Verification items for the finished model (mm, model axes). A direction names the side the tool comes from. Coordinates: 2 decimals unless noted, no trailing zeros. Order: outer loops, then holes, each group sorted by start corner. A loop starts at its lowest first (then second) coordinate and runs counter-clockwise, first axis right, second up. Notation, with made-up numbers: M 21,0 L 73,0 A15 ccw 73,14 Z; hole C 89,89.5 d3. An arc over 180 degrees is marked long. Write item = value, one per line.
```python
from build123d import *

# Parameters (mm, degrees)
EXTRUDE_577_DEPTH                       = 10
EXTRUDE_START                           = 3
EXTRUDE_1331_DEPTH                      = 2
FILLET_1_R                              = 1
EXTRUDE_2001_DEPTH                      = 6
EXTRUDE_2001_DEPTH_BACK                 = 9
CUT_EXTRUDE_2109_REACH                  = 26.775
CUT_EXTRUDE_2109_END_RADIUS             = 7.25
SKETCH_6_R                              = 1.75
CUT_EXTRUDE_2109_DIRECTION_2_REACH      = 26.775
CUT_EXTRUDE_2109_DIRECTION_2_END_RADIUS = 10.75
SKETCH_7_R                              = 1.4
EXTRUDE_2720_DEPTH                      = 2
EXTRUDE_2720_2_DEPTH                    = 2
CHAMFER_2_SIZE                          = 1.5
EXTRUDE_START_2                         = 1
EXTRUDE_3078_DEPTH                      = 1
CHAMFER_3_SIZE                          = 1.5
CHAMFER_4_SIZE                          = 4.5
CHAMFER_4_SIZE2                         = 0.5


# Some blends are built 0.0001 mm under size
with BuildPart() as part:
    # Эскиз1 → Extrude 577 (new body)
    with BuildSketch(Plane.XY):
        with BuildLine():
            ThreePointArc((-5.712121212, 4.464770012), (0, -7.25), (5.712121212, 4.464770012))
            ThreePointArc((5.712121212, 4.464770012), (5.884169654, 5.868479146), (7.287878788, 5.696430705))
            ThreePointArc((7.287878788, 5.696430705), (0, -9.25), (-7.287878788, 5.696430705))
            ThreePointArc((-7.287878788, 5.696430705), (-5.884169654, 5.868479146), (-5.712121212, 4.464770012))
        make_face()
    extrude(amount=EXTRUDE_577_DEPTH)

    # Эскиз5 → Extrude 2001 (add, two sides: drawn at the far end of the back side and taken through both)
    with BuildSketch(Plane.XY.offset(10).offset(-EXTRUDE_2001_DEPTH_BACK)):
        with BuildLine():
            ThreePointArc((-5.058139535, -5.194008514), (0, -7.25), (5.058139535, -5.194008514))
            ThreePointArc((5.058139535, -5.194008514), (7.532795961, -5.226804475), (7.5, -7.7014609))
            ThreePointArc((7.5, -7.7014609), (0, -10.75), (-7.5, -7.7014609))
            ThreePointArc((-7.5, -7.7014609), (-7.532795961, -5.226804475), (-5.058139535, -5.194008514))
        make_face()
    extrude(amount=EXTRUDE_2001_DEPTH + EXTRUDE_2001_DEPTH_BACK)

    # Cut-Extrude 2109: up to this cylinder (the profile starts outside it)
    cut_extrude_2109_end = Plane(origin=(0, 0, 12), z_dir=(0, 0, -1)) * Cylinder(CUT_EXTRUDE_2109_END_RADIUS, 69.05, mode=Mode.PRIVATE)
    # Эскиз6 → Cut-Extrude 2109 (cut, up to the surface)
    with BuildSketch(Plane(origin=(0, -9.25, 0), x_dir=(-1, 0, 0), z_dir=(0, -1, 0)), mode=Mode.PRIVATE) as cut_extrude_2109_sk1:
        with Locations(Location((0, -12, 0), (0, 0, 270))):
            Circle(SKETCH_6_R)
    cut_extrude_2109_tool1 = extrude(cut_extrude_2109_sk1.sketch, amount=-CUT_EXTRUDE_2109_REACH, mode=Mode.PRIVATE) - cut_extrude_2109_end
    add(cut_extrude_2109_tool1.solids().sort_by_distance((0, -9.25, 12))[0], mode=Mode.SUBTRACT)

    # Cut-Extrude 2109 direction 2: up to this cylinder (the profile starts inside it)
    cut_extrude_2109_direction_2_end = Plane(origin=(0, 0, 12), z_dir=(0, 0, 1)) * Cylinder(CUT_EXTRUDE_2109_DIRECTION_2_END_RADIUS, 76.05, mode=Mode.PRIVATE)
    # Эскиз6 → Cut-Extrude 2109 direction 2 (cut, up to the surface)
    with BuildSketch(Plane(origin=(0, -9.25, 0), x_dir=(-1, 0, 0), z_dir=(0, -1, 0)), mode=Mode.PRIVATE) as cut_extrude_2109_direction_2_sk1:
        with Locations(Location((0, -12, 0), (0, 0, 270))):
            Circle(SKETCH_6_R)
    cut_extrude_2109_direction_2_tool1 = extrude(cut_extrude_2109_direction_2_sk1.sketch, amount=CUT_EXTRUDE_2109_DIRECTION_2_REACH, mode=Mode.PRIVATE) & cut_extrude_2109_direction_2_end
    add(cut_extrude_2109_direction_2_tool1.solids().sort_by_distance((0, -9.25, 12))[0], mode=Mode.SUBTRACT)

    # Фаска2
    chamfer_2_edges = [part.edges().sort_by_distance(p)[0] for p in [
        (-8.027867462, -6.512593205, 1),
        (8.027867462, -6.512593205, 1),
        (0, -10.75, 1),
    ]]
    chamfer(chamfer_2_edges, length=CHAMFER_2_SIZE - 0.0001)  # a hair under: the kernel refuses the full size



with BuildPart() as body_2:
    # Эскиз3 → Extrude 1331 (new body)
    with BuildSketch(Plane(origin=(0, 0, 0), x_dir=(-1, 0, 0), z_dir=(0, 0, -1)).offset(EXTRUDE_START)):
        with BuildLine():
            Line((-1.5, 7.09313048), (-2.75, 0.004028205))
            ThreePointArc((-2.75, 0.004028205), (-3.918577626, -3.728601804), (-6, -7.04006392))
            ThreePointArc((-6, -7.04006392), (0, -9.25), (6, -7.04006392))
            ThreePointArc((6, -7.04006392), (3.918577626, -3.728601804), (2.75, 0.004028205))
            Line((2.75, 0.004028205), (1.5, 7.09313048))
            ThreePointArc((1.5, 7.09313048), (0, 7.25), (-1.5, 7.09313048))
        make_face()
    extrude(amount=-EXTRUDE_1331_DEPTH)

    # Скругление1
    # the kernel refuses this fillet: 1 mm, written as the material it takes off along each edge
    with BuildSketch(Plane(origin=(-17.735965382, 2.646458234, -3), x_dir=(0.6567344577177726, -0.7541219079473445, 0), z_dir=(-0.7541219079473445, -0.6567344577177726, 0))) as fillet_1_piece_1:
        with BuildLine():
            CenterArc((15.217148054 + FILLET_1_R, FILLET_1_R), FILLET_1_R, 180, 90)
            Line((15.217148054 + FILLET_1_R, 0), (15.217148054, 0))
            Line((15.217148054, 0), (15.217148054, FILLET_1_R))
        make_face()
    revolve(axis=Axis((-17.735965382, 2.646458234, -3), (0, 0, 1)), revolution_arc=38.948703068, mode=Mode.SUBTRACT)
    with BuildSketch(Plane(origin=(-2.75, 0.004028205, -3), x_dir=(0, 0, 1), z_dir=(0.17364817766693094, 0.984807753012208, 0)), Plane(origin=(1.065879556, 9.555149862, -3), x_dir=(0, 0, 1), z_dir=(0.1736481776669306, -0.984807753012208, 0))) as fillet_1_piece_2:
        with BuildLine():
            CenterArc((FILLET_1_R, FILLET_1_R), FILLET_1_R, 180, 90)
            Line((0, FILLET_1_R), (0, 0))
            Line((0, 0), (FILLET_1_R, 0))
        make_face()
    extrude(amount=9.698463104, mode=Mode.SUBTRACT)
    with BuildSketch(Plane(origin=(17.735965382, 2.646458234, -3), x_dir=(-0.9848077530122082, -0.17364817766692925, 0), z_dir=(-0.17364817766692925, 0.9848077530122082, 0))) as fillet_1_piece_3:
        with BuildLine():
            CenterArc((15.217148054 + FILLET_1_R, FILLET_1_R), FILLET_1_R, 180, 90)
            Line((15.217148054 + FILLET_1_R, 0), (15.217148054, 0))
            Line((15.217148054, 0), (15.217148054, FILLET_1_R))
        make_face()
    revolve(axis=Axis((17.735965382, 2.646458234, -3), (0, 0, 1)), revolution_arc=38.948703068, mode=Mode.SUBTRACT)


with BuildPart() as body_3:
    # Эскиз7 → Extrude 2720 (new body)
    with BuildSketch(Plane(origin=(0, 0, -3), x_dir=(-1, 0, 0), z_dir=(0, 0, -1))):
        with BuildLine():
            Line((-7.059505235, -8.866162387), (-5.204391621, -7.647013002))
            ThreePointArc((-5.204391621, -7.647013002), (-3.557692308, -8.538461538), (-1.765200931, -9.080009123))
            Line((-1.765200931, -9.080009123), (-1.324605701, -11.255703859))
            ThreePointArc((-1.324605701, -11.255703859), (-6.442307692, -15.461538462), (-7.059505235, -8.866162387))
        make_face()
        with Locations((-5, -12)):
            Circle(SKETCH_7_R, mode=Mode.SUBTRACT)
    extrude(amount=-EXTRUDE_2720_DEPTH)


with BuildPart() as body_4:
    # Эскиз7 → Extrude 2720 2 (new body)
    with BuildSketch(Plane(origin=(0, 0, -3), x_dir=(-1, 0, 0), z_dir=(0, 0, -1))):
        with BuildLine():
            Line((1.324605701, -11.255703859), (1.765200931, -9.080009123))
            ThreePointArc((1.765200931, -9.080009123), (3.557692308, -8.538461538), (5.204391621, -7.647013002))
            Line((5.204391621, -7.647013002), (7.059505235, -8.866162387))
            ThreePointArc((7.059505235, -8.866162387), (6.442307692, -15.461538462), (1.324605701, -11.255703859))
        make_face()
        with Locations(Location((5, -12, 0), (0, 0, 180))):
            Circle(SKETCH_7_R, mode=Mode.SUBTRACT)
    extrude(amount=-EXTRUDE_2720_2_DEPTH)


with BuildPart() as part_1:
    add(part.part)

    add(body_2.part)  # Extrude 3078 merges body 2

    add(body_3.part)  # Extrude 3078 merges body 3

    add(body_4.part)  # Extrude 3078 merges body 4
    # Эскиз8 → Extrude 3078 (add)
    with BuildSketch(Plane(origin=(0, 0, 0), x_dir=(-1, 0, 0), z_dir=(0, 0, -1)).offset(EXTRUDE_START_2)):
        with BuildLine():
            ThreePointArc((-6, -7.04006392), (0, -9.25), (6, -7.04006392))
            ThreePointArc((6, -7.04006392), (5.386302599, -6.244403593), (4.826454597, -5.409975603))
            ThreePointArc((4.826454597, -5.409975603), (0, -7.25), (-4.826454597, -5.409975603))
            ThreePointArc((-4.826454597, -5.409975603), (-5.386302599, -6.244403593), (-6, -7.04006392))
        make_face()
    extrude(amount=-EXTRUDE_3078_DEPTH)

    # Фаска3
    chamfer_3_edges = [part_1.edges().sort_by_distance(p)[0] for p in [
        (6.4, -12, -1),
        (-6.4, -12, -1),
    ]]
    chamfer(chamfer_3_edges, length=CHAMFER_3_SIZE)

    # Фаска4
    chamfer_4_edges = [part_1.edges().sort_by_distance(p)[0] for p in [
        (0, 7.25, -1),
    ]]
    chamfer_4_side = [part_1.faces().sort_by_distance(p)[0] for p in [
        (0, -1.121169898, -1),
    ]]
    chamfer(chamfer_4_edges, length=CHAMFER_4_SIZE, length2=CHAMFER_4_SIZE2, reference=chamfer_4_side[0])


solid = part_1.part
```
Item 1: Sectioned sample at C-C, the plane y = 1.25. Give the number of separate pieces and of enclosed holes in the cut face, then the cut area to 3 significant figures.
Report:
separate_pieces = 3
enclosed_holes = 0
area = 50.2 mm^2
Item 2: Sectioned sample at B-B, the plane z = 12. Enter the section's corners in (x, y), then the cut area to 3 significant figures.
Report:
outline = M -7.5,-7.7 A10.75 ccw -1.75,-10.61 L -1.75,-7.04 A7.25 cw -5.06,-5.19 A1.75 ccw Z; M 1.75,-10.61 A10.75 ccw 7.5,-7.7 A1.75 ccw 5.06,-5.19 A7.25 cw 1.75,-7.04 Z
area = 45.9 mm^2
Item 3: Release check for a two-part mould opening along Y. For faces 4 (the cylindrical face through (-1.81, 3.602, -2.715)), 5 (the cylindrical face through (-5.9, 5.88, 4.93)), 6 (the cylindrical face through (0.12, -10.75, 9.16)) record: pulls with the +Y half, pulls with the -Y half, needs draft (parallel to the pull), parting line crosses it, or undercut.
Report:
face_4 = pulls with the +Y half
face_5 = undercut
face_6 = pulls with the -Y half
Item 4: Gauge pin test, flat ends, axial feed: pin 1 (1.3 mm diameter, centred on x = 7, y = 1.5, fed in from +Z); pin 2 (1.3 mm diameter, centred on x = 8, y = -2, fed in from -Z); pin 3 (2.5 mm diameter, centred on x = 5, y = -12, fed in from -Z); pin 4 (2 mm diameter, centred on x = -3, y = -13.5, fed in from +Z). Record the tip position at first contact, or that the pin passes through.
Report:
pin_1 = 10
pin_2 = 0
pin_3 = through
pin_4 = -1
Item 5: Sectioned sample at A-A, the plane y = -12. Enter the section's corners in (x, z).
Report:
outline = M -8.75,-3 L -6.4,-3 L -6.4,-2.5 L -7.9,-1 L -8.75,-1 Z; M -3.6,-3 L -1.25,-3 L -1.25,-1 L -2.1,-1 L -3.6,-2.5 Z; M 1.25,-3 L 3.6,-3 L 3.6,-2.5 L 2.1,-1 L 1.25,-1 Z; M 6.4,-3 L 8.75,-3 L 8.75,-1 L 7.9,-1 L 6.4,-2.5 Z
Item 6: Tool access check on faces 1 (the flat face through (-6.12, -8.25, -2.01)), 2 (the flat face through (0, -8, 16)), 3 (the cylindrical face through (7.859, -5.694, 10.655)). Record the directions out of +Z, -Z, +X, -X, +Y, -Y that give a thin tool (end or side, any length) a straight path to the whole face; none if there is none.
Report:
face_1 = -Z, -X
face_2 = +Z, +X, -X, +Y, -Y
face_3 = +Z
Item 7: Scan lines: L1, parallel to Z at x = 7.5, y = 4; L2, parallel to X at y = 0, z = 7; L3, parallel to X at y = 5.5, z = 2.5. Record each from-to range of solid material in increasing order. Write a range as from..to.
Report:
L1 = 0..10
L2 = -9.25..-7.25, 7.25..9.25
L3 = -7.44..-5.59, 5.59..7.44
